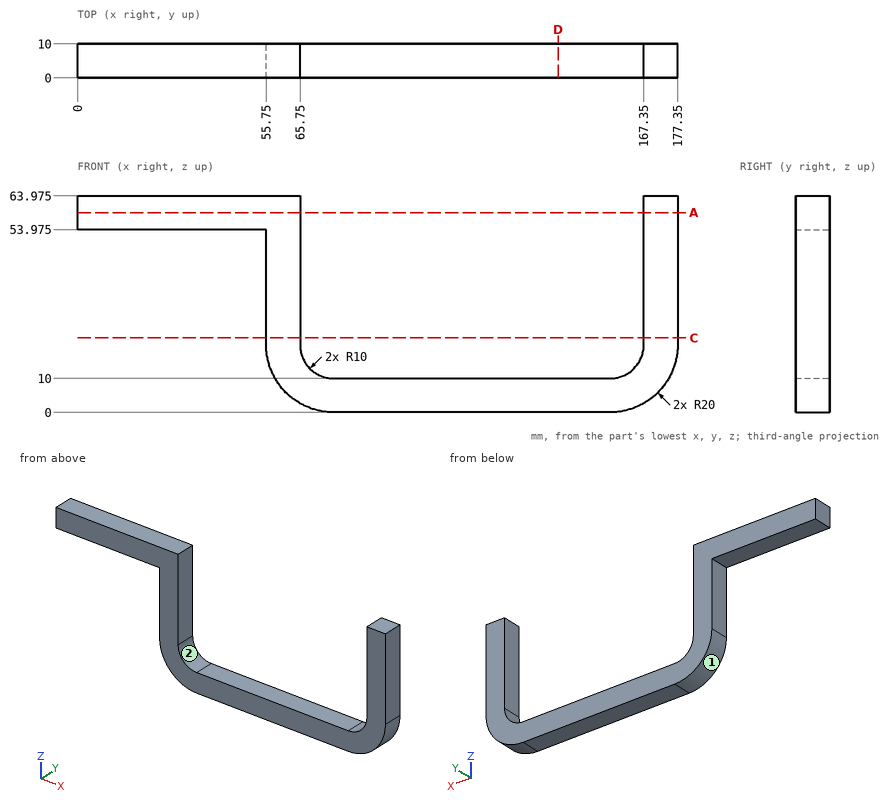
Geometry: see drawing. Coordinates: mm, zero at the bounding-box minimum. A direction names the side the tool comes from. Round coordinates to 2 decimals unless told otherwise and drop trailing zeros. Order: outer loops, then holes, each group sorted by start corner. A loop starts at its lowest first (then second) coordinate and runs counter-clockwise, first axis right, second up. Notation, with made-up numbers: (80.5, 15) -> (137.5, 15) arc R18 ccw to (137.5, 28) -> close; hole circle Ø6 at (27, 14). An arc over 180 degrees is marked (long way). Use CSV: the item, a comma, the result in double quotes.
(1) Ray query, L1, parallel to X at y = 1.75, z = 37; L2, parallel to Z at x = 115, y = 6.25; L3, parallel to X at y = 5.25, z = 19 (1 decimal). Return the intervals inside material, ascending.
Report:
L1,"55.75 to 65.75, 167.35 to 177.35"
L2,"0 to 10"
L3,"55.8 to 65.8, 167.3 to 177.3"
(2) Section C-C on z = 22. Return the cut outline in (x, y).
Report:
outline,"(55.75, 0) -> (65.75, 0) -> (65.75, 10) -> (55.75, 10) -> close; (167.35, 0) -> (177.35, 0) -> (177.35, 10) -> (167.35, 10) -> close"
(3) Access query for the marked faces 1 and 2. Directions: +Z, -Z, +X, -X, +Y, -Y. A direction counts if a zero-diameter tool reaches every point of the face in a straight line with its end or side. Return the directions, or none.
Report:
face 1,"-Z, -X, +Y, -Y"
face 2,"+Z, +Y, -Y"
(4) Section A-A on z = 59. Return the cut outline in (x, y).
Report:
outline,"(0, 0) -> (65.75, 0) -> (65.75, 10) -> (0, 10) -> close; (167.35, 0) -> (177.35, 0) -> (177.35, 10) -> (167.35, 10) -> close"
(5) Section D-D on x = 142. Return the cut outline in (y, z).
Report:
outline,"(0, 0) -> (10, 0) -> (10, 10) -> (0, 10) -> close"
(6) First-contact query: pin 1 Ø5 at (x, y) = (33.5, 2.5) entering from -Z (3 decimals); pin 2 Ø5 at (y, z) = (7, 40.5) entering from -X; pin 3 Ø1 at (y, z) = (4, 11) entering from +X. Flat tips, straight axial feed; report the tip coordinate or a pass-through.
Report:
pin 1,"z = 53.975"
pin 2,"x = 55.75"
pin 3,"x = 175.45"
